```python
from build123d import *

# Parameters (mm, degrees)
F0_R     = 1.5
F0_R_2   = 1
F0_R_3   = 2
F0_R_4   = 3
F1_DEPTH = 2.5
F2_R     = 2.6
F3_DEPTH = 1


with BuildPart() as f1:
    # F0 (on Right) → F1 (new body)
    with BuildSketch(Plane.YZ):
        with BuildLine():
            ThreePointArc((-24.764499, 8.807669), (-20.91644, 5.130545), (-19.5, 0))
            Line((-19.5, 0), (-15.5, 0))
            Line((-15.5, 0), (-15.5, 3))
            Line((-15.5, 3), (-16.75, 3))
            Line((-16.75, 3), (-16.75, 7.5))
            Line((-16.75, 7.5), (-11.25, 7.5))
            Line((-11.25, 7.5), (-11.25, 3))
            Line((-11.25, 3), (-12.5, 3))
            Line((-12.5, 3), (-12.5, 0))
            Line((-12.5, 0), (-3, 0))
            Line((-3, 0), (-3, -2.5))
            Line((-3, -2.5), (5, -2.5))
            Line((5, -2.5), (5, 0))
            Line((5, 0), (10, 0))
            Line((10, 0), (10, 3))
            Line((10, 3), (8.75, 3))
            Line((8.75, 3), (8.75, 7.5))
            Line((8.75, 7.5), (14.25, 7.5))
            Line((14.25, 7.5), (14.25, 3))
            Line((14.25, 3), (13, 3))
            Line((13, 3), (13, 0))
            Line((13, 0), (19.5, 0))
            Line((19.5, 0), (19.730406, 2.430542))
            ThreePointArc((19.730406, 2.430542), (20.102681, 3.905521), (20.901261, 5.200289))
            Line((20.901261, 5.200289), (29.029949, 14.74632))
            ThreePointArc((29.029949, 14.74632), (29.828529, 16.041087), (30.200804, 17.516067))
            Line((30.200804, 17.516067), (30.450974, 20.155105))
            ThreePointArc((30.450974, 20.155105), (30.22612, 20.886698), (29.549811, 21.245015))
            Line((29.549811, 21.245015), (23.576589, 21.811254))
            ThreePointArc((23.576589, 21.811254), (22.22397, 22.52789), (21.774261, 23.991074))
            Line((21.774261, 23.991074), (21.955369, 25.901569))
            ThreePointArc((21.955369, 25.901569), (20.886782, 31.430613), (17, 35.505553))
            Line((17, 35.505553), (-3, 47.052559))
            ThreePointArc((-3, 47.052559), (-30.769889, 42.239762), (-31.017419, 14.056993))
            Line((-31.017419, 14.056993), (-30.763877, 13.747545))
            ThreePointArc((-30.763877, 13.747545), (-28.006432, 10.983406), (-24.764499, 8.807669))
        make_face()
        with Locations((-25, 13.024149)):
            Circle(F0_R, mode=Mode.SUBTRACT)
        with Locations((-8.660254, 23.185045)):
            Circle(F0_R, mode=Mode.SUBTRACT)
        with BuildLine():
            ThreePointArc((-2.962619, 26.440837), (-2.404462, 28.48741), (-0.357889, 27.929254))
            ThreePointArc((-0.357889, 27.929254), (0.890951, 22.725413), (-0.85181, 17.665537))
            ThreePointArc((-0.85181, 17.665537), (-2.942522, 17.306479), (-3.30158, 19.397191))
            ThreePointArc((-3.30158, 19.397191), (-2.105582, 22.869615), (-2.962619, 26.440837))
        make_face(mode=Mode.SUBTRACT)
        with Locations((16.28461, 13.024149)):
            Circle(F0_R, mode=Mode.SUBTRACT)
        with BuildLine():
            ThreePointArc((23.104724, 16.833569), (22.20356, 17.923479), (23.29347, 18.824643))
            Line((23.29347, 18.824643), (26.280081, 18.541524))
            ThreePointArc((26.280081, 18.541524), (27.181244, 17.451614), (26.091335, 16.55045))
            Line((26.091335, 16.55045), (23.104724, 16.833569))
        make_face(mode=Mode.SUBTRACT)
        with Locations((-29.874508, 26)):
            Circle(F0_R_2, mode=Mode.SUBTRACT)
        with Locations((-29.716234, 31)):
            Circle(F0_R_3, mode=Mode.SUBTRACT)
        with Locations((-26.622516, 37.832197)):
            Circle(F0_R_4, mode=Mode.SUBTRACT)
        with Locations((-20.755296, 42.503999)):
            Circle(F0_R_3, mode=Mode.SUBTRACT)
        with Locations((-4.5, 43.299782)):
            Circle(F0_R, mode=Mode.SUBTRACT)
        with Locations((-15.755296, 43.903425)):
            Circle(F0_R_2, mode=Mode.SUBTRACT)
        with Locations((16.28461, 31.299782)):
            Circle(F0_R, mode=Mode.SUBTRACT)
    extrude(amount=F1_DEPTH)

    # F2 (on face) → F3 (cut)
    with BuildSketch(Plane(origin=(0, 0, 0), x_dir=(0, -1, 0), z_dir=(-1, 0, 0))):
        with Locations((4.5, 43.299782)):
            Circle(F2_R)
        with Locations((-16.28461, 31.299782)):
            Circle(F2_R)
        with Locations((-16.28461, 13.024149)):
            Circle(F2_R)
        with Locations((25, 13.024149)):
            Circle(F2_R)
    extrude(amount=-F3_DEPTH, mode=Mode.SUBTRACT)


solid = f1.part
```
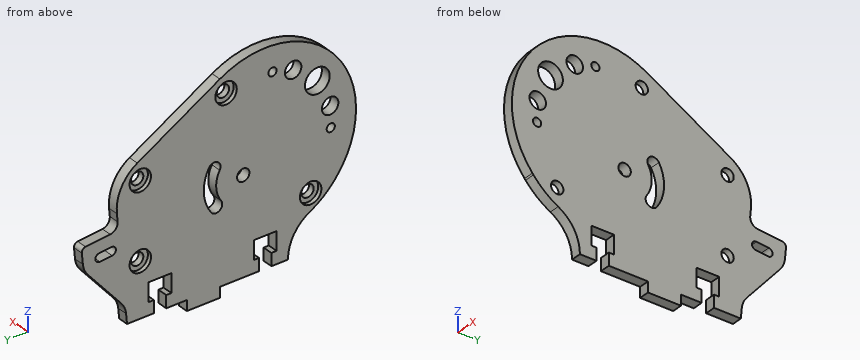
Check sheet for the modelled part. Datum: model origin and axes. Units: mm. Give positions to 0.01 mm unless a question says otherwise; leave off trailing zeros. Order: outer loops, then holes, each group sorted by start corner. A loop starts at its lowest first (then second) coordinate and runs counter-clockwise, first axis right, second up. Notation, with made-up numbers: (-3.5, 75.5) -> (36.5, 75.5) arc R23 cw to (36.5, 91.5) -> close; hole circle Ø2 at (-10, 78). An arc over 180 degrees is marked (long way). Use CSV: the item, a comma, the result in double quotes. Start each with the question number.
1) Sectioned sample at C-C, the plane x = 1.8. Give the number of separate pieces and of enclosed holes in the cut face, plus the area to 3 significant figures.
2) Material ranges on line 1 (Y direction, x = 0.6, z = 41); line 2 (Z direction, x = 0.2, y = -25); line 3 (Z direction, x = 2.3, y = -31.5), recorded low to high. Write a range as from..to.
3) Sectioned sample at B-B, the plane y = -4.5. Record the boundary of the cut face in (x, z), plus the area to 3 significant figures.
4) Sectioned sample at A-A, the plane z = 39.5. Record the boundary of the cut face in (x, y) (3 decimals), plus the area to 3 significant figures.
5) Go/stop test with flat-tipped pins: P1, Ø4, axis at y = -4.5, z = 43.3, coming from the -X side; P2, Ø2.5, axis at y = -4.5, z = 43.5, coming from the -X side; P3, Ø10, axis at y = 13, z = 12, coming from the -X side; P4, Ø1.2, axis at x = 1.5, y = 16.5, coming from the -Z side. Record where each tip stops, or that it passes through.
Recorded:
1,separate pieces,"1"
1,enclosed holes,"12"
1,area,"2,220 mm2"
2,line 1,"-31.75..-22.07, -19.44..-5.71, -3.29..7.48"
2,line 2,"8.94..10.42, 15.62..35.31, 40.36..47.05"
2,line 3,"14.67..30.1, 31.9..41.33"
3,outline,"(0, 0) -> (2.5, 0) -> (2.5, 41.8) -> (1, 41.8) -> (1, 40.7) -> (0, 40.7) -> close; (0, 45.9) -> (1, 45.9) -> (1, 44.8) -> (2.5, 44.8) -> (2.5, 47.84) -> (0, 47.84) -> close"
3,area,"110 mm2"
4,outline,"(0, -32.755) -> (2.5, -32.755) -> (2.5, -29.116) -> (0, -29.116) -> close; (0, -24.129) -> (2.5, -24.129) -> (2.5, 10.081) -> (0, 10.081) -> close"
4,area,"94.6 mm2"
5,P1,"x = 1"
5,P2,"through"
5,P3,"x = 0"
5,P4,"z = 0"
